Could you check a few things on this drawing? It's one solid part, dimensions in mm from its lowest x, y, z. A direction names the side the tool comes from. Round coordinates to 2 decimals unless told otherwise and drop trailing zeros. Write each loop counter-clockwise with the first axis right and the second up, starting at its lowest first coordinate (ties: lowest second). Pieces come first, ordered by that corner, then holes. Notation, with made-up numbers: (62, 39) - (82, 39) arc R26 cw to (82, 72) - close; hole circle Ø7 at (22, 24.5). An arc over 180 degrees is marked (long way). Put each result on its own line as item: value.
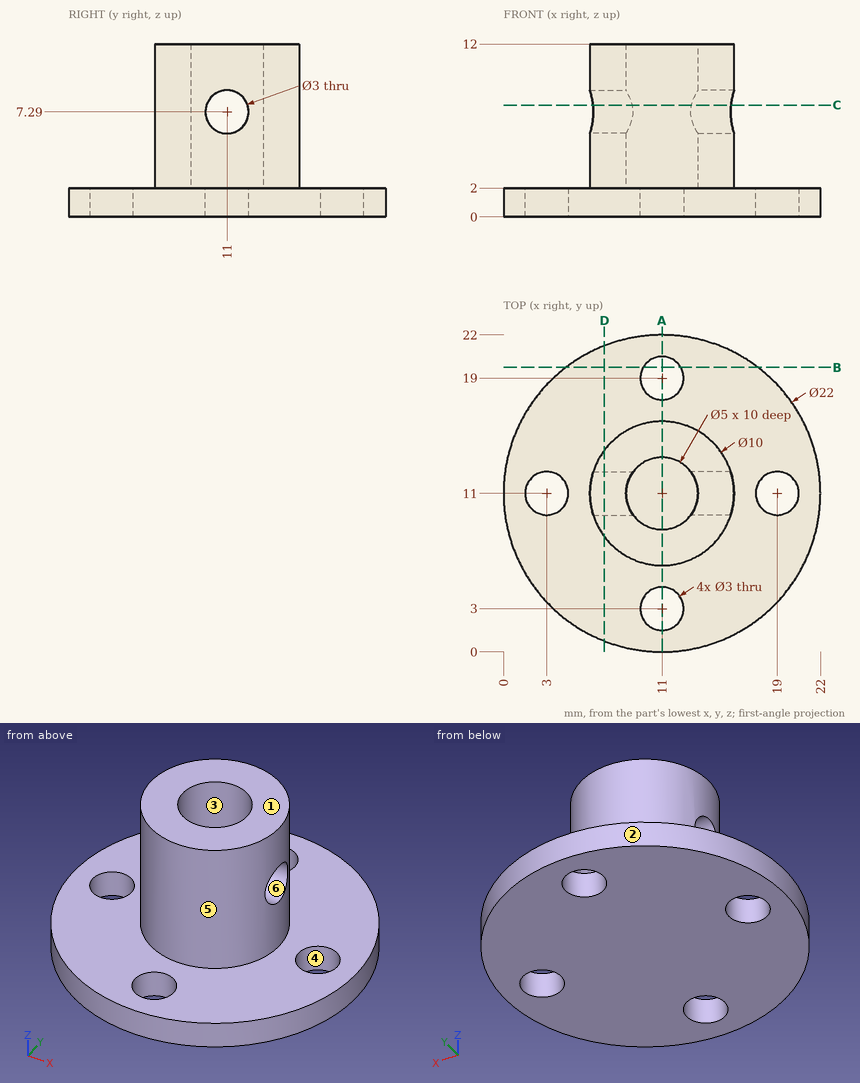
(1) Imagine slicing it at D-D, the plane x = 7. List the corners of the cut face in (y, z) for me.
Values found:
outline: (0.75, 0) - (21.25, 0) - (21.25, 2) - (14, 2) - (14, 12) - (8, 12) - (8, 2) - (0.75, 2) - close; hole circle Ø3 at (11, 7.29)
(2) Imagine slicing it at C-C, the plane z = 7.75. List the corners of the cut face in (x, y) for me, then the cut area to 3 significant figures.
Values found:
outline: (6.21, 9.57) arc R5 ccw to (15.79, 9.57) - (13.05, 9.57) arc R2.5 cw to (8.95, 9.57) - close; (6.21, 12.43) - (8.95, 12.43) arc R2.5 cw to (13.05, 12.43) - (15.79, 12.43) arc R5 ccw to start
area: 44.2 mm^2
(3) If we mould it in two halves opening along Y, with no side actions, what happens to the marked faces 1, 2, 3 and 4? For each: pulls with the +Y half, pulls with the -Y half, needs draft (parallel to the pull), parting line crosses it, or undercut.
Values found:
face 1: needs draft
face 2: parting line crosses it
face 3: undercut
face 4: undercut
(4) For the marked faces 5 and 6, which set-ups out of +Z, -Z, +X, -X, +Y, -Y let a thin tool reach every point of the face, with its end or its side?
Values found:
face 5: +Z
face 6: +X, -X
(5) Please list where these lines run through material, in increasing order: probe 1 along Y at (x, z) = (11, 0.9); probe 2 along Y at (x, z) = (11, 4); probe 3 along X at (y, z) = (13, 3.75) (1 decimal). Write a range as from..to.
Values found:
probe 1: y = 0..1.5, 4.5..17.5, 20.5..22
probe 2: y = 6..8.5, 13.5..16
probe 3: x = 6.4..9.5, 12.5..15.6
(6) Imagine slicing it at B-B, the plane y = 19.75. List the corners of the cut face in (x, z) for me.
Values found:
outline: (4.33, 0) - (9.7, 0) - (9.7, 2) - (4.33, 2) - close; (12.3, 0) - (17.67, 0) - (17.67, 2) - (12.3, 2) - close
(7) Imagine slicing it at A-A, the plane x = 11. List the corners of the cut face in (y, z) for me.
Values found:
outline: (0, 0) - (1.5, 0) - (1.5, 2) - (0, 2) - close; (4.5, 0) - (17.5, 0) - (17.5, 2) - (16, 2) - (16, 12) - (13.5, 12) - (13.5, 2) - (8.5, 2) - (8.5, 12) - (6, 12) - (6, 2) - (4.5, 2) - close; (20.5, 0) - (22, 0) - (22, 2) - (20.5, 2) - close
(8) I'm going to push flat-ended pins straight in: pin 1 (3.5 mm diameter, centred on y = 11, z = 7.29, fed in from +X); pin 2 (4 mm diameter, centred on x = 11, y = 3, fed in from +Z); pin 3 (4 mm diameter, centred on y = 7, z = 9, fed in from -X). Where does each tip first touch, or does it pass through?
Values found:
pin 1: stops at x = 16
pin 2: stops at z = 2
pin 3: stops at x = 6.42
